For this review, use the dimensioned drawing (mm, ordinates from the lowest corner) and the shaded views. Give positions to 0.01 mm unless a question says otherwise; leave off trailing zeros. Write each loop counter-clockwise with the first axis right and the second up, starting at its lowest first coordinate (ties: lowest second). Pieces come first, ordered by that corner, then holes. Notation, with made-up numbers: (82, -35.75) -> (127, -35.75) arc R22 ccw to (127, -10.75) -> close; hole circle Ø5 at (-32.5, -12.5). An arc over 180 degrees is marked (long way). Answer as CSV lines item,"result".
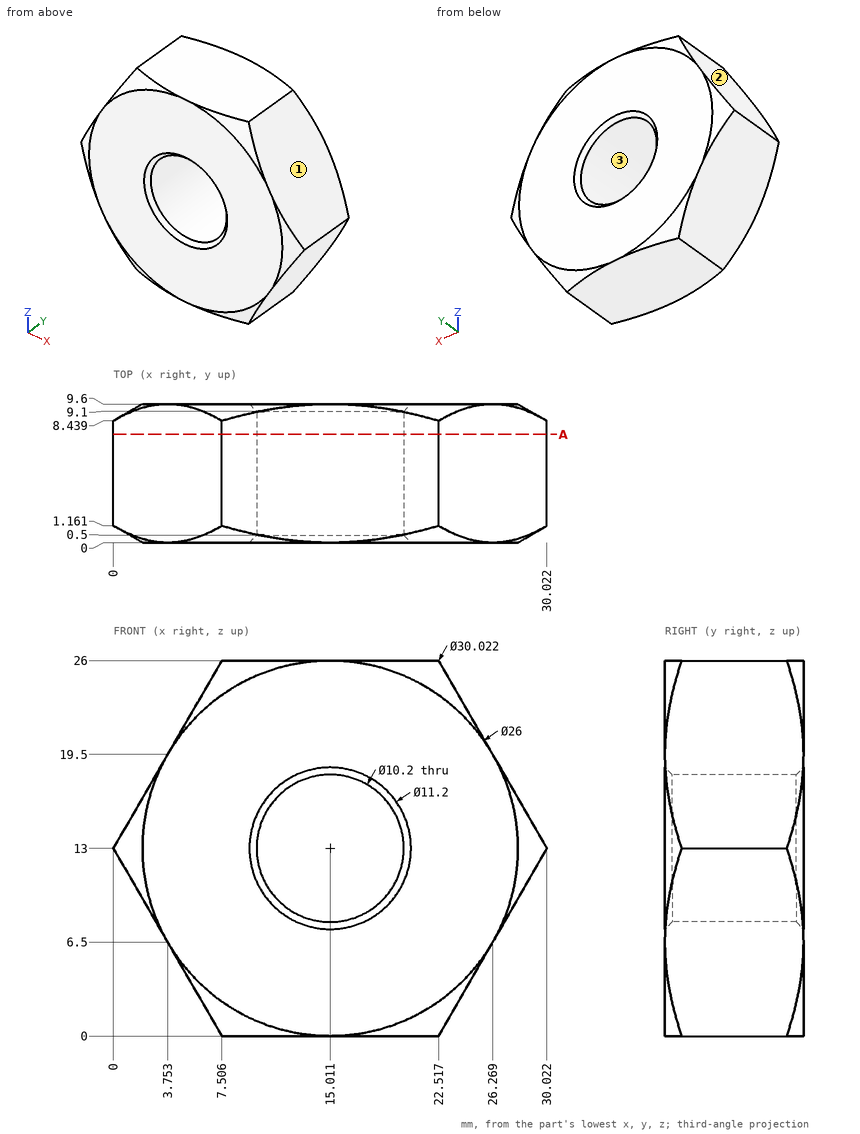
Q1. Draft analysis for pull direction X (two halves, no side actions). For the marked faces 1, 2 and 3, state which applies: released by +X, released by -X, zero draft, split by the parting line, or undercut.
Answer block:
face 1,"released by +X"
face 2,"released by -X"
face 3,"undercut"
Q2. To check wall thickness, follow probe 1 along Z at (x, y) = (13, 1); probe 2 along Z at (x, y) = (16.5, 4); probe 3 along X at (y, z) = (8.5, 10.5) (1 decimal). State the ranges of each line that lie inside material, in increasing order. Write a range as [from, to].
Answer block:
probe 1,"z = [0, 8.31], [17.69, 26]"
probe 2,"z = [0, 8.12], [17.88, 26]"
probe 3,"x = [1.4, 10.6], [19.5, 28.6]"
Q3. Clearance check with flat-ended pins moving along their axes: pin 1 (3 mm diameter, centred on y = 3.5, z = 4, fed in from -X); pin 2 (3 mm diameter, centred on y = 4.5, z = 21, fed in from -X); pin 3 (2 mm diameter, centred on y = 1, z = 17.5, fed in from -X); pin 4 (4 mm diameter, centred on x = 17.5, z = 17.5, fed in from -Y). State where each tip first meets the part, or that it passes through.
Answer block:
pin 1,"stops at x = 4.33"
pin 2,"stops at x = 3.75"
pin 3,"stops at x = 2.02"
pin 4,"stops at y = 0"
Q4. Add section A-A (y = 7.5). Write out the cut boundary in (x, z) (1 decimal), plus the area to 3 significant figures.
Answer block:
outline,"(0, 13) -> (7.5, 0) -> (22.5, 0) -> (30, 13) -> (22.5, 26) -> (7.5, 26) -> close; hole circle Ø10.2 at (15, 13)"
area,"504 mm2"
